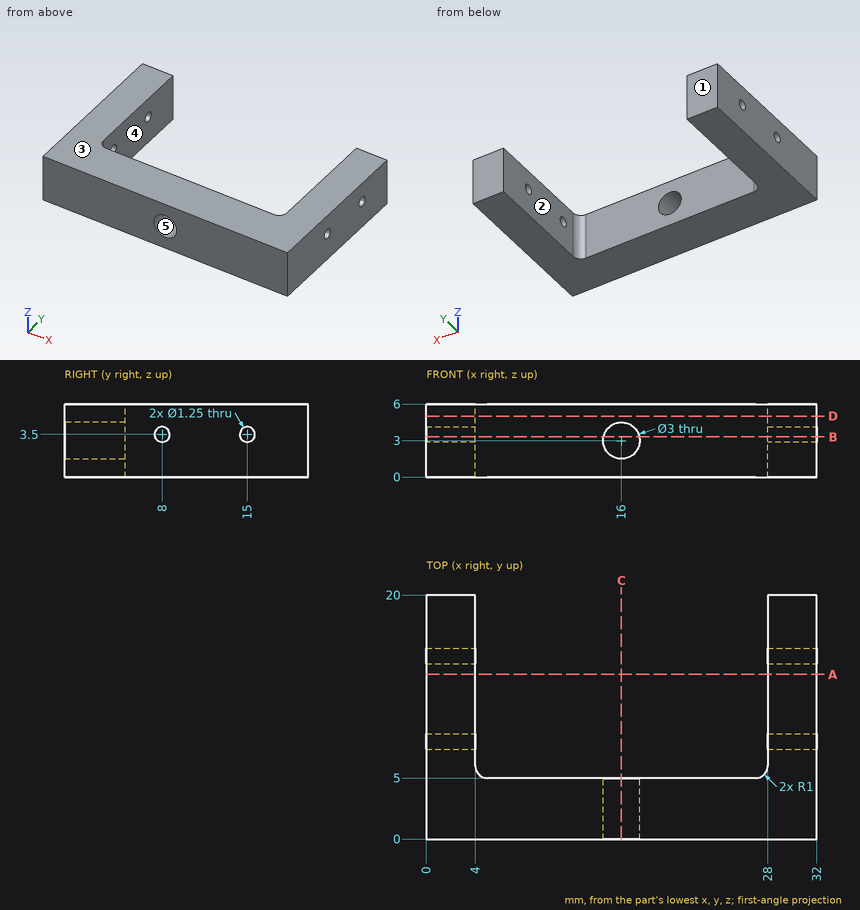
Here's the drawing with two shaded views (mm, measured from the low corner). I have some questions. A direction names the side the tool comes from. Round coordinates to 2 decimals unless told otherwise and drop trailing zeros. Loops run counter-clockwise (first coordinate to the right, second up) from the corner with the lowest first, then second, coordinate; pieces in that order, holes last. Notation, with made-up numbers: M 48,51.25 L 66,51.25 A27 ccw 66,81.25 Z; hole C -31,75.5 d5. An arc over 180 degrees is marked long. Put each result on its own line as item: value.
Q1. Imagine slicing it at C-C (x = 16). Write out the boundary of the cut face in (y, z), then the cut area to 3 significant figures.
Check result:
outline: M 0,0 L 5,0 L 5,1.5 L 0,1.5 Z; M 0,4.5 L 5,4.5 L 5,6 L 0,6 Z
area: 15.0 mm2
Q2. For pin 1 (1 mm diameter, centred on x = 24.5, z = 2, fed in from -Y); pin 2 (3 mm diameter, centred on x = 14, z = 4.5, fed in from +Y), each with a flat end and sliding along its axis, tell me the tip position at first contact or that it passes through.
Check result:
pin 1: y = 0
pin 2: y = 5
Q3. Imagine slicing it at A-A (y = 13.5). Write out the boundary of the cut face in (x, z), then the cut area to 3 significant figures.
Check result:
outline: M 0,0 L 4,0 L 4,6 L 0,6 Z; M 28,0 L 32,0 L 32,6 L 28,6 Z
area: 48.0 mm2
Q4. On a 3-axis mill with a long thin cutter (end or side, diameter ignored), from which of +Z, -Z, +X, -X, +Y, -Y can I reach the whole of each face in a straight line? I mean the marked faces 1 and 2. Say none if no direction works.
Check result:
face 1: +Z, -Z, +X, -X, +Y
face 2: +Z, -Z, +Y
Q5. Imagine slicing it at D-D (z = 5). Write out the boundary of the cut face in (x, y), then the cut area to 3 significant figures.
Check result:
outline: M 0,0 L 32,0 L 32,20 L 28,20 L 28,6 A1 cw 27,5 L 5,5 A1 cw 4,6 L 4,20 L 0,20 Z
area: 280 mm2
Q6. Imagine slicing it at B-B (z = 3.3). State how many separate pieces and enclosed holes the cut face has, then the cut area to 3 significant figures.
Check result:
separate pieces: 6
enclosed holes: 0
area: 247 mm2
Q7. Thinking about a two-plate mould opening in Z: for the marked faces 3, 4 and 5, which applies, released by +Z, released by -Z, zero draft, split by the parting line, or undercut?
Check result:
face 3: released by +Z
face 4: zero draft
face 5: undercut
Q8. I need wall thicknesses on probe 1 along Y at (x, z) = (30.45, 3.5) (3 decimals); probe 2 along X at (y, z) = (17, 0.8); probe 3 along X at (y, z) = (1.6, 3). Which ranges of each line are inside material? Lowest first, please.
Check result:
probe 1: 0 to 7.375, 8.625 to 14.375, 15.625 to 20
probe 2: 0 to 4, 28 to 32
probe 3: 0 to 14.5, 17.5 to 32
